Geometry check sheet. Reference: the model listing, model coordinates, mm. Face numbers are marked on the shaded views. A direction names the side the tool comes from. Give positions to 0.01 mm unless a question says otherwise; leave off trailing zeros. Write each loop counter-clockwise with the first axis right and the second up, starting at its lowest first coordinate (ties: lowest second). Pieces come first, ordered by that corner, then holes. Notation, with made-up numbers: (-20.5, 61.5) -> (37.5, 61.5) arc R24 ccw to (37.5, 79.5) -> close; hole circle Ø7 at (33, -11). An arc over 180 degrees is marked (long way). Write item = value, one per line. Start each with the question number.
1. Thickness scan on line 1 along Z through (x, y) = (-4.75, -1.35); line 2 along X through (y, z) = (-0.15, 13); line 3 along X through (y, z) = (0.2, -4). Record the ranges inside material, lowest first.
2. Cross-section at A-A, the plane y = -1.05. Record the cut outline in (x, z).
3. Depth check by flat-ended pin: P1, Ø6, axis at x = -7.5, z = -9, coming from the -Y side; P2, Ø2, axis at y = 2, z = 1.5, coming from the -X side; P3, Ø3, axis at y = -1.5, z = -2, coming from the -X side; P4, Ø1, axis at x = -5, y = -1.5, coming from the -Z side. Enter the tip coordinate at first touch or a pass-through.
4. Set-up check for the marked faces 1, 2, 3 and 4: record each of +Z, -Z, +X, -X, +Y, -Y from which the full face is reachable in a straight line by a thin tool's end or side.
5. Cross-section at B-B, the plane z = 12. Record the cut outline in (x, y), plus the area to 3 significant figures.
```python
from build123d import *

# Parameters (mm, degrees)
SKETCH_1_R      = 3
EXTRUDE_1_DEPTH = 16
SKETCH_2_W      = 10.054460063
SKETCH_2_H      = 4.37386331
EXTRUDE_2_DEPTH = 5
CHAMFER_1_SIZE  = 8


with BuildPart() as part:
    # 스케치1 → 보스-돌출1 (new, symmetric)
    with BuildSketch(Plane.XY):
        Circle(SKETCH_1_R)
    extrude(amount=EXTRUDE_1_DEPTH, both=True)

    # 스케치2 → 보스-돌출2 (add, symmetric)
    with BuildSketch(Plane.XY):
        with Locations((-5.027230032, 0.110464554)):
            Rectangle(SKETCH_2_W, SKETCH_2_H)
    extrude(amount=EXTRUDE_2_DEPTH, both=True)

    # 모따기1
    chamfer_1_edges = [part.edges().sort_by_distance(p)[0] for p in [
        (-10.054460063, 0.110464554, 5),
    ]]
    chamfer(chamfer_1_edges, length=CHAMFER_1_SIZE)


solid = part.part
```
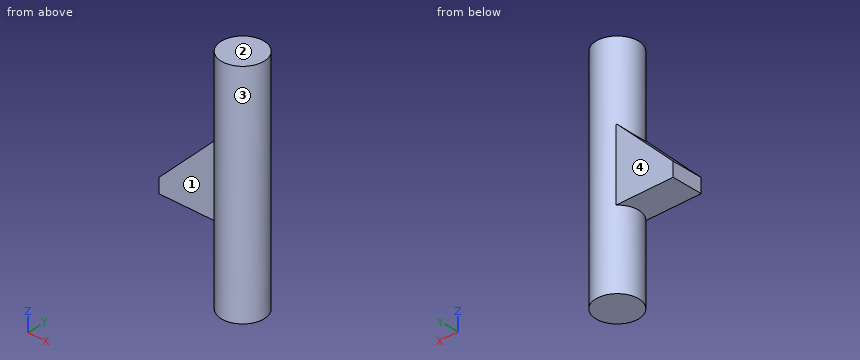
Answers:
q1.line_1 = -5 to 2.3
q1.line_2 = -3 to 3
q1.line_3 = -10.05 to 2.99
q2.outline = (-10.05, -5) -> (-2.81, -5) -> (-2.81, -16) -> (2.81, -16) -> (2.81, 16) -> (-2.81, 16) -> (-2.81, 4.24) -> (-10.05, -3) -> close
q3.P1 = through
q3.P2 = -6.55
q3.P3 = -10.05
q3.P4 = -5
q4.face_1 = +Z, -Z, -X, -Y
q4.face_2 = +Z, +X, -X, +Y, -Y
q4.face_3 = none
q4.face_4 = +Z, -Z, -X, +Y
q5.outline = circle Ø6 at (0, 0)
q5.area = 28.3 mm^2
